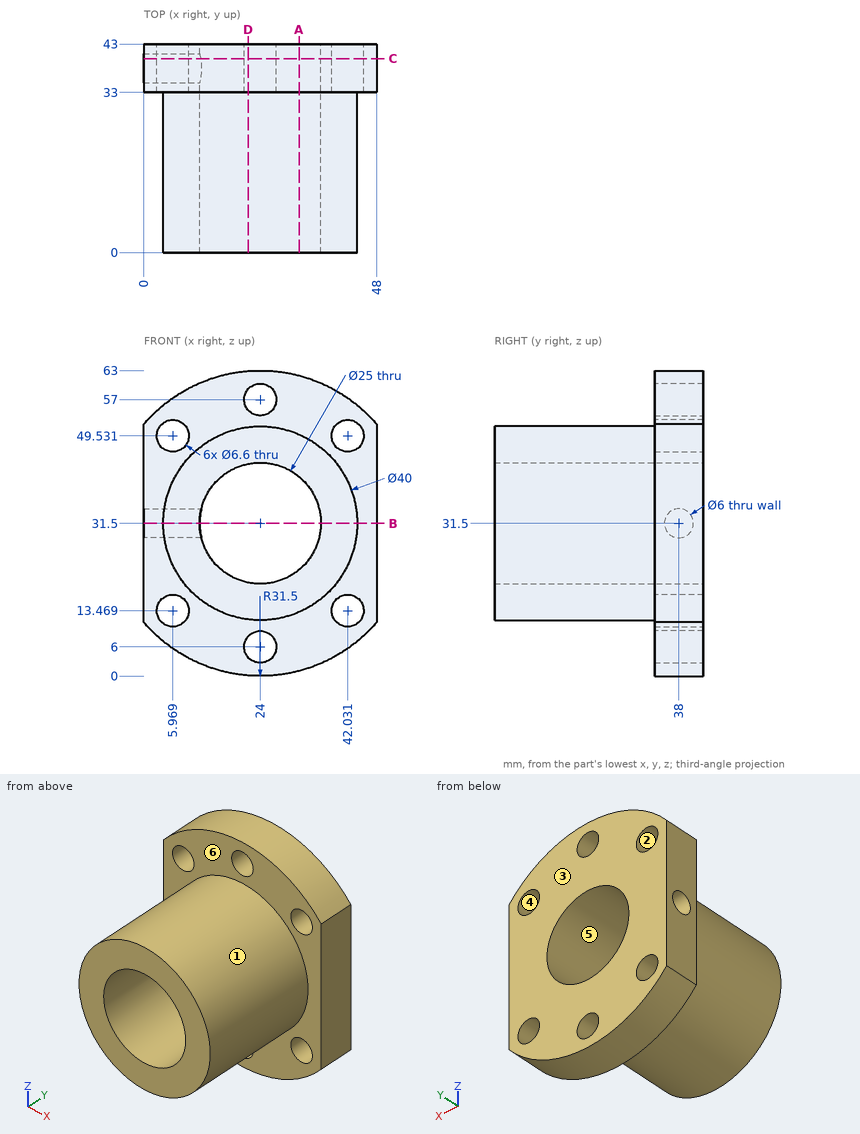
Study the drawing (mm; zero at the part's minimum x, y, z) and answer. A direction names the side the tool comes from. Coordinates: 2 decimals unless noted, no trailing zeros. Write each loop counter-clockwise with the first axis right and the second up, starting at its lowest first coordinate (ties: lowest second). Pieces come first, ordered by that corner, then holes.
Q1. Which of the six approach directions +Z, -Z, +X, -X, +Y, -Y give full straight-line access (tool end or side, diameter ignored) to the marked faces 5 and 6?
Returned:
face 5: +Y, -Y
face 6: -Y
Q2. Find the intervals of material crossed by line 1 along Z through (x, y) = (24.5, 21); line 2 along Y through (x, z) = (17.5, 60.5); line 3 along X through (y, z) = (32, 21), in increasing order.
Returned:
line 1: z = 11.51 to 19.01, 43.99 to 51.49
line 2: y = 33 to 43
line 3: x = 6.98 to 17.22, 30.78 to 41.02
Q3. Section D-D, the plane x = 21.5 is taken. Write down the section's boundary in (y, z), then the cut area to 3 significant figures.
Returned:
outline: (0, 11.66) - (33, 11.66) - (33, 8.15) - (43, 8.15) - (43, 19.25) - (0, 19.25) - close; (0, 43.75) - (43, 43.75) - (43, 54.85) - (33, 54.85) - (33, 51.34) - (0, 51.34) - close; (33, 0.1) - (43, 0.1) - (43, 3.85) - (33, 3.85) - close; (33, 59.15) - (43, 59.15) - (43, 62.9) - (33, 62.9) - close
area: 798 mm2
Q4. Section C-C, the plane y = 40 is taken. Write down the section's boundary in (x, z).
Returned:
outline: (0, 11.1) arc R31.5 ccw to (48, 11.1) - (48, 51.9) arc R31.5 ccw to (0, 51.9) - (0, 33.74) - (11.7, 33.74) arc R12.5 cw (long way) to (11.7, 29.26) - (0, 29.26) - close; hole circle Ø6.6 at (5.97, 13.47); hole circle Ø6.6 at (5.97, 49.53); hole circle Ø6.6 at (24, 6); hole circle Ø6.6 at (24, 57); hole circle Ø6.6 at (42.03, 13.47); hole circle Ø6.6 at (42.03, 49.53)
Q5. Given P1, Ø12, axis at y = 16, z = 24, coming from the -X side; P2, Ø9.5, axis at y = 38, z = 31.5, coming from the -X side; P3, Ø1.5, axis at x = 25.5, y = 32.5, coming from the +Z side; P4, Ø5, axis at x = 13.5, y = 22, coming from the -Z side, each flat-ended and moving along its own axis, determine where each tip first touches the part or whether it passes through.
Returned:
P1: stops at x = 4.06
P2: stops at x = 0
P3: stops at z = 62.99
P4: stops at z = 13.17
Q6. Section A-A, the plane x = 32 is taken. Write down the section's boundary in (y, z) (1 decimal).
Returned:
outline: (0, 13.2) - (33, 13.2) - (33, 1) - (43, 1) - (43, 21.9) - (0, 21.9) - close; (0, 41.1) - (43, 41.1) - (43, 62) - (33, 62) - (33, 49.8) - (0, 49.8) - close
Q7. Section B-B, the plane z = 31.5 is taken. Write down the section's boundary in (x, y).
Returned:
outline: (0, 33) - (4, 33) - (4, 0) - (11.5, 0) - (11.5, 35) - (0, 35) - close; (0, 41) - (11.5, 41) - (11.5, 43) - (0, 43) - close; (36.5, 0) - (44, 0) - (44, 33) - (48, 33) - (48, 43) - (36.5, 43) - close
Q8. The mould has two halves that part along X. Classify the marked faces 1, 2, 3 and 4: released by +X, released by -X, zero draft, split by the parting line, or undercut.
Returned:
face 1: split by the parting line
face 2: undercut
face 3: zero draft
face 4: undercut
